Input: part model. Units: mm. Frame: model coordinates. Face numbers are marked on the shaded views. A direction names the side the tool comes from. Give positions to 0.01 mm unless a question says otherwise; leave off trailing zeros. Write each loop counter-clockwise with the first axis right and the second up, starting at its lowest first coordinate (ties: lowest second). Pieces come first, ordered by that corner, then holes.
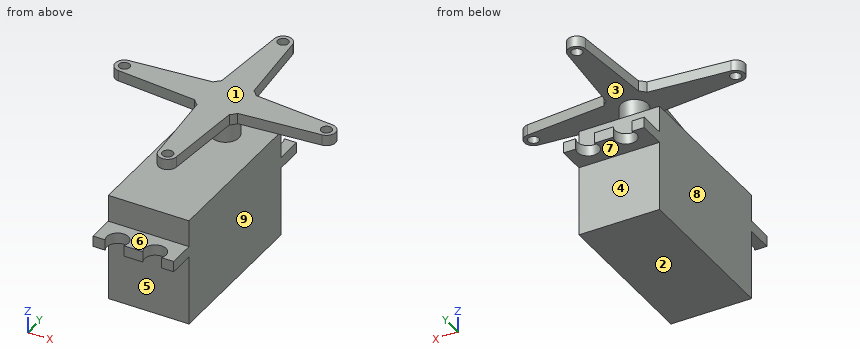
```python
from build123d import *

# Parameters (mm, degrees)
F0_W      = 19.05
F0_H      = 38.1
F1_DEPTH  = 16.51
F2_W      = 19.05
F2_H      = 50.8
F3_DEPTH  = 2.54
F4_R      = 2.54
F5_DEPTH  = 2.54
F6_W      = 19.05
F6_H      = 38.1
F7_DEPTH  = 6.35
F8_R      = 3.175
F9_DEPTH  = 6.35
F10_R     = 6.35
F11_DEPTH = 2.54
F12_R     = 1.27
F13_DEPTH = 2.54


with BuildPart() as f1:
    # F0 (on Top) → F1 (new body)
    with BuildSketch(Plane.XY):
        with Locations((-35.5894370005, 14.3955526778)):
            Rectangle(F0_W, F0_H)
    extrude(amount=F1_DEPTH)

    # F2 (on face) → F3 (join)
    with BuildSketch(Plane.XY.offset(16.51)):
        with Locations((-35.5894370005, 14.3955526778)):
            Rectangle(F2_W, F2_H)
    extrude(amount=F3_DEPTH)

    # F4 (on face) → F5 (cut)
    with BuildSketch(Plane.XY.offset(19.05)):
        with Locations((-40.0344370005, 38.5255526778)):
            Circle(F4_R)
        with Locations((-31.1444370005, 38.5255526778)):
            Circle(F4_R)
        with Locations((-31.1444370005, -9.7344473222)):
            Circle(F4_R)
        with Locations((-40.0344370005, -9.7344473222)):
            Circle(F4_R)
    extrude(amount=-F5_DEPTH, mode=Mode.SUBTRACT)

    # F6 (on face) → F7 (join)
    with BuildSketch(Plane.XY.offset(19.05)):
        with Locations((-35.5894370005, 14.3955526778)):
            Rectangle(F6_W, F6_H)
    extrude(amount=F7_DEPTH)

    # F8 (on face) → F9 (join)
    with BuildSketch(Plane.XY.offset(25.4)):
        with Locations((-35.5894370005, 27.0955526778)):
            Circle(F8_R)
    extrude(amount=F9_DEPTH)

    # F10 (on face) → F11 (join)
    with BuildSketch(Plane.XY.offset(31.75)):
        with Locations((-35.5894370005, 27.0955526778)):
            Circle(F10_R)
    extrude(amount=F11_DEPTH)

    # F12 (on face) → F13 (join)
    with BuildSketch(Plane.XY.offset(34.29)):
        with BuildLine():
            Line((-37.7391201011, 51.1530616765), (-39.3994370005, 32.1755526778))
            ThreePointArc((-39.3994370005, 32.1755526778), (-35.5894370005, 33.4455526778), (-31.7794370005, 32.1755526778))
            Line((-31.7794370005, 32.1755526778), (-33.4397538998, 51.1530616765))
            ThreePointArc((-33.4397538998, 51.1530616765), (-35.5894370005, 53.1228833158), (-37.7391201011, 51.1530616765))
        make_face()
        with Locations((-35.5894370005, 50.964988775)):
            Circle(F12_R, mode=Mode.SUBTRACT)
        with BuildLine():
            Line((-11.5319280018, 29.2452357785), (-30.5094370005, 30.9055526778))
            ThreePointArc((-30.5094370005, 30.9055526778), (-29.2394370005, 27.0955526778), (-30.5094370005, 23.2855526778))
            Line((-30.5094370005, 23.2855526778), (-11.5319280018, 24.9458695772))
            ThreePointArc((-11.5319280018, 24.9458695772), (-9.5621063624, 27.0955526778), (-11.5319280018, 29.2452357785))
        make_face()
        with Locations((-11.7200009033, 27.0955526778)):
            Circle(F12_R, mode=Mode.SUBTRACT)
        with BuildLine():
            Line((-33.4397538998, 3.0380436792), (-31.7794370005, 22.0155526778))
            ThreePointArc((-31.7794370005, 22.0155526778), (-35.5894370005, 20.7455526778), (-39.3994370005, 22.0155526778))
            Line((-39.3994370005, 22.0155526778), (-37.7391201011, 3.0380436792))
            ThreePointArc((-37.7391201011, 3.0380436792), (-35.5894370005, 1.0682220398), (-33.4397538998, 3.0380436792))
        make_face()
        with Locations((-35.5894370005, 3.2261165806)):
            Circle(F12_R, mode=Mode.SUBTRACT)
        with BuildLine():
            ThreePointArc((-40.6694370005, 23.2855526778), (-41.9394370005, 27.0955526778), (-40.6694370005, 30.9055526778))
            Line((-40.6694370005, 30.9055526778), (-59.6469459991, 29.2452357785))
            ThreePointArc((-59.6469459991, 29.2452357785), (-61.6167676385, 27.0955526778), (-59.6469459991, 24.9458695772))
            Line((-59.6469459991, 24.9458695772), (-40.6694370005, 23.2855526778))
        make_face()
        with Locations((-59.4588730976, 27.0955526778)):
            Circle(F12_R, mode=Mode.SUBTRACT)
    extrude(amount=-F13_DEPTH)


solid = f1.part
```
Q1. Mould query, pull axis Z, two halves, no side actions, for the marked faces 1, 2, 3 and 4. Classes: +Z half, -Z half, draft (parallel to the pull), parting line (faces both ways), or undercut.
Q2. Access query for the marked faces 5, 6, 7, 8 and 9. Directions: +Z, -Z, +X, -X, +Y, -Y. A direction counts if a zero-diameter tool reaches every point of the face in a straight line with its end or side. Return the directions, or none.
Q3. Section D-D, the plane z = 8.5. Return the cut outline in (x, y).
Q4. Section A-A, the plane y = 17.5. Return the cut outline in (x, z), then the cut area to 3 significant figures.
Q5. Pin query (flat end, axial travel): pin 1 (1.9 mm diameter, centred on x = -31, y = 38, fed in from -Z); pin 2 (5 mm diameter, centred on x = -31, y = -7, fed in from +Z); pin 3 (1.5 mm diameter, centred on y = -2, z = 5, fed in from +X); pin 4 (4.5 mm diameter, centred on x = -40.03, y = 38.53, fed in from -Z). Return the tip coordinate at first contact, or that it passes through.
Q6. Section B-B, the plane x = -27.5. Return the cut outline in (y, z), then the cut area to 3 significant figures.
Q7. Material intervals for line 1 along Z through (x, y) = (-36, 8); line 2 along Z through (x, y) = (-35, 35); line 3 along Y through (x, z) = (-11.72, 33.15), sorted ascending.
Q8. Section C-C, the plane y = 34.5. Return the cut outline in (x, z), then the cut area to 3 significant figures.
Solutions:
1. face 1: +Z half
1. face 2: -Z half
1. face 3: undercut
1. face 4: draft
2. face 5: -Z, +X, -X, -Y
2. face 6: +Z, +X, -X, -Y
2. face 7: -Z, +X, -X, +Y
2. face 8: -Z, -X, +Y, -Y
2. face 9: -Z, +X, +Y, -Y
3. outline: (-45.11, -4.65) - (-26.06, -4.65) - (-26.06, 33.45) - (-45.11, 33.45) - close
4. outline: (-45.11, 0) - (-26.06, 0) - (-26.06, 25.4) - (-45.11, 25.4) - close; (-39, 31.75) - (-32.17, 31.75) - (-32.17, 34.29) - (-39, 34.29) - close
4. area: 501 mm2
5. pin 1: passes through
5. pin 2: stops at z = 25.4
5. pin 3: stops at x = -26.06
5. pin 4: stops at z = 31.75
6. outline: (-11, 16.51) - (-4.65, 16.51) - (-4.65, 0) - (33.45, 0) - (33.45, 16.51) - (39.8, 16.51) - (39.8, 19.05) - (33.45, 19.05) - (33.45, 25.4) - (-4.65, 25.4) - (-4.65, 19.05) - (-11, 19.05) - close; (23.55, 31.75) - (30.64, 31.75) - (30.64, 34.29) - (23.55, 34.29) - close
6. area: 1,020 mm2
7. line 1: z = 0 to 25.4, 31.75 to 34.29
7. line 2: z = 16.51 to 19.05, 31.75 to 34.29
7. line 3: y = 24.93 to 25.83, 28.37 to 29.26
8. outline: (-45.11, 16.51) - (-26.06, 16.51) - (-26.06, 19.05) - (-45.11, 19.05) - close; (-39.2, 31.75) - (-31.98, 31.75) - (-31.98, 34.29) - (-39.2, 34.29) - close
8. area: 66.7 mm2
